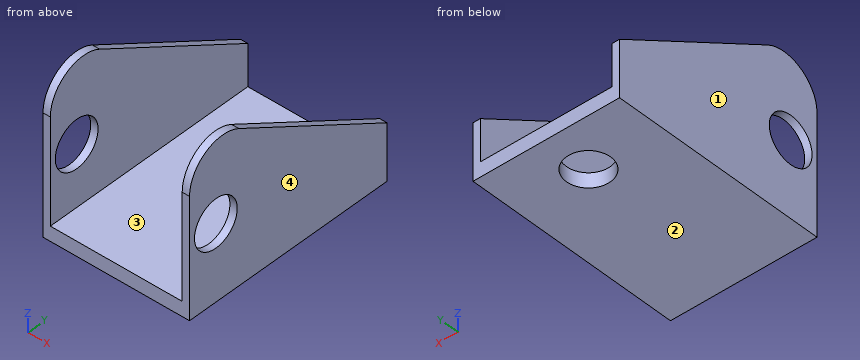
from build123d import *

# Parameters (mm, degrees)
SKETCH1_W           = 20
SKETCH1_H           = 30
BOSS_EXTRUDE1_DEPTH = 2
BOSS_EXTRUDE2_DEPTH = 1
LPATTERN1_COUNT     = 2
LPATTERN1_PITCH     = 19
FILLET1_R           = 5
FILLET2_R           = 5
SKETCH3_R           = 3.25
CUT_EXTRUDE1_DEPTH  = 33.869206831
SKETCH4_R           = 3
CUT_EXTRUDE2_DEPTH  = 28.935367507


with BuildPart() as part:
    # Sketch1 → Boss-Extrude1 (new body)
    with BuildSketch(Plane.XY):
        Rectangle(SKETCH1_W, SKETCH1_H)
    extrude(amount=BOSS_EXTRUDE1_DEPTH)

    # Sketch2 → Boss-Extrude2 (add)
    with BuildSketch(Plane(origin=(10, 0, 0), x_dir=(0, 0, -1), z_dir=(1, 0, 0))):
        Polygon((-2, 15), (-7.679491924, 15), (-25, -15), (-2, -15), align=None)
    boss_extrude2 = extrude(amount=-BOSS_EXTRUDE2_DEPTH)

    # LPattern1: Boss-Extrude2 ×2
    with Locations(*[(-i * LPATTERN1_PITCH, 0, 0) for i in range(1, LPATTERN1_COUNT)]):
        add(boss_extrude2)

    # Fillet1
    fillet1_edges = [part.edges().sort_by_distance(p)[0] for p in [
        (-9.5, -15, 25),
    ]]
    fillet(fillet1_edges, radius=FILLET1_R)

    # Fillet2
    fillet2_edges = [part.edges().sort_by_distance(p)[0] for p in [
        (9.5, -15, 25),
    ]]
    fillet(fillet2_edges, radius=FILLET2_R)

    # Sketch3 → Cut-Extrude1 (cut, through all)
    with BuildSketch(Plane.ZY.offset(10)):
        with Locations((10.339745962, -11)):
            Circle(SKETCH3_R)
    extrude(amount=-CUT_EXTRUDE1_DEPTH, mode=Mode.SUBTRACT)

    # Sketch4 → Cut-Extrude2 (cut, through all)
    with BuildSketch(Plane(origin=(0, 0, 0), x_dir=(-1, 0, 0), z_dir=(0, 0, -1))):
        with Locations((0, 8.588876522)):
            Circle(SKETCH4_R)
    extrude(amount=-CUT_EXTRUDE2_DEPTH, mode=Mode.SUBTRACT)


solid = part.part
Part model, mm, in its own coordinate system. Face numbers are marked on the shaded views. Round coordinates to 2 decimals unless told otherwise and drop trailing zeros. Loops run counter-clockwise (first coordinate to the right, second up) from the corner with the lowest first, then second, coordinate; pieces in that order, holes last. Notation, with made-up numbers: (66.5, 53.25) - (99.5, 53.25) arc R28 cw to (99.5, 92.25) - close; hole circle Ø11 at (-11, 35.5). An arc over 180 degrees is marked (long way). Answer as a JSON object with one key per item and string values.
Item 1: Band-saw the part on C-C on y = -12. List the corners of the cut face in (x, z), plus the area to 3 significant figures.
Output:
{"outline": "(-10, 0) - (10, 0) - (10, 7.25) - (9, 7.25) - (9, 2) - (-9, 2) - (-9, 7.25) - (-10, 7.25) - close; (-10, 13.43) - (-9, 13.43) - (-9, 20.92) - (-10, 20.92) - close; (9, 13.43) - (10, 13.43) - (10, 20.92) - (9, 20.92) - close", "area": "65.5 mm2"}
Item 2: Band-saw the part on D-D on z = 9.25. List the corners of the cut face in (x, y).
Output:
{"outline": "(-10, -15) - (-9, -15) - (-9, -14.06) - (-10, -14.06) - close; (-10, -7.94) - (-9, -7.94) - (-9, 12.28) - (-10, 12.28) - close; (9, -15) - (10, -15) - (10, -14.06) - (9, -14.06) - close; (9, -7.94) - (10, -7.94) - (10, 12.28) - (9, 12.28) - close"}
Item 3: Band-saw the part on B-B on z = 2.5. List the corners of the cut face in (x, y).
Output:
{"outline": "(-10, -15) - (-9, -15) - (-9, 15) - (-10, 15) - close; (9, -15) - (10, -15) - (10, 15) - (9, 15) - close"}
Item 4: Wall check: L1, parallel to X at y = -9, z = 13.75; L2, parallel to Y at x = 0, z = 1.3; L3, parallel to Z at x = -1, y = -7.5. Give the ranges that are in metal, low to high.
Output:
{"L1": "-10 to -9, 9 to 10", "L2": "-15 to 5.59, 11.59 to 15", "L3": "0 to 2"}
Item 5: Pin check, flat tip, straight feed: pin 1 (3 mm diameter, centred on x = -7, y = -1.5, fed in from +Z). Stop position of the tip, or through.
Output:
{"pin 1": "z = 2"}
Item 6: Band-saw the part on A-A on x = 0. List the corners of the cut face in (y, z).
Output:
{"outline": "(-15, 0) - (5.59, 0) - (5.59, 2) - (-15, 2) - close; (11.59, 0) - (15, 0) - (15, 2) - (11.59, 2) - close"}
Item 7: Pull direction X, two halves, no side cores. Call the marked faces 1, 2, 3 and 4: pulls with the +X half, pulls with the -X half, needs draft (parallel to the pull), parting line crosses it, or undercut.
Output:
{"face 1": "pulls with the -X half", "face 2": "needs draft", "face 3": "undercut", "face 4": "pulls with the +X half"}
